Part print with two shaded views. Sizes in mm from the minimum x, y, z corner. A direction names the side the tool comes from. Give positions to 0.01 mm unless a question says otherwise; leave off trailing zeros. Loops run counter-clockwise (first coordinate to the right, second up) from the corner with the lowest first, then second, coordinate; pieces in that order, holes last. Notation, with made-up numbers: M 44.25,-0.75 L 72.25,-0.75 A21 cw 72.25,4.25 Z; hole C 43.25,23 d10. An arc over 180 degrees is marked long. Answer in a Markdown table with one row per item.
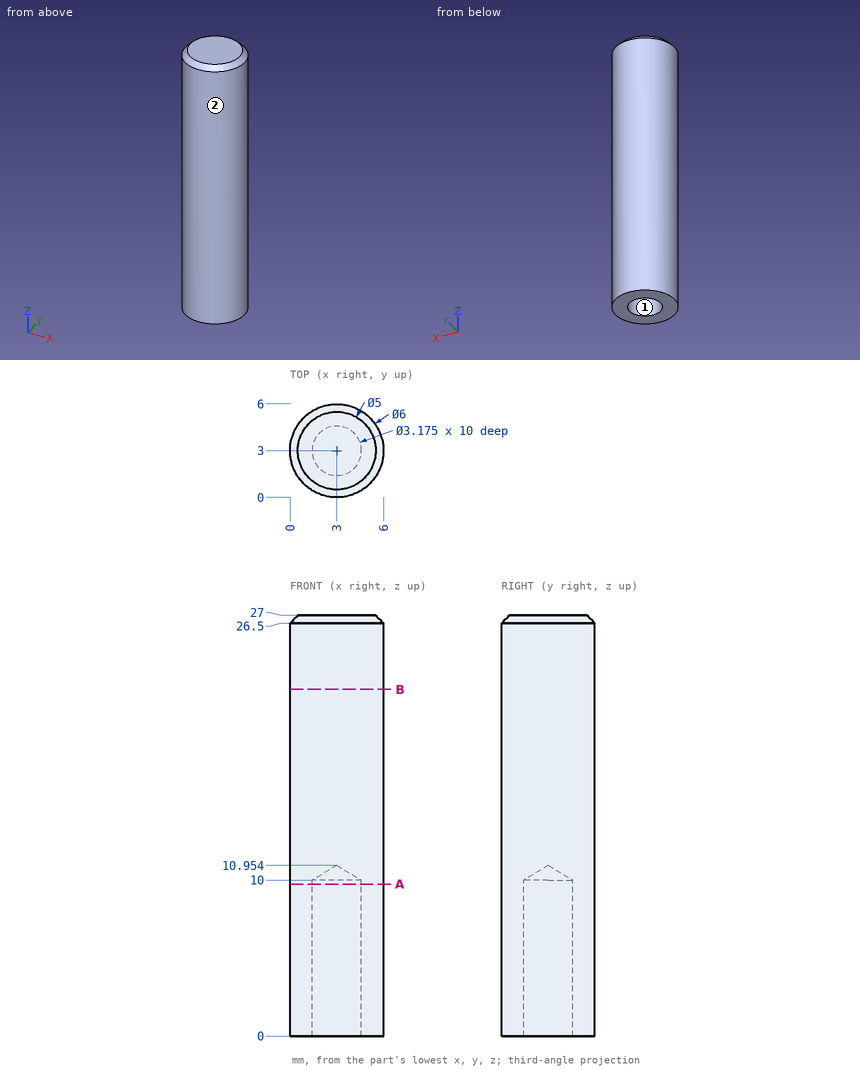
Q1. Probe probe 1 along X at (y, z) = (3.1, 8); probe 2 along Y at (x, z) = (3, 3); probe 3 along X at (y, z) = (2.85, 18.75). List the from-to ranges inside material, lowest first.
Reported:
| item | result |
|---|---|
| probe 1 | 0 to 1.42, 4.58 to 6 |
| probe 2 | 0 to 1.41, 4.59 to 6 |
| probe 3 | 0 to 6 |
Q2. Saw through at B-B (z = 22.25). Give the cut face in (x, y).
Reported:
| item | result |
|---|---|
| outline | C 3,3 d6 |
Q3. 3-axis set-ups, long thin cutter, end or side, ignore diameter. For the marked faces 1 and 2: which of +Z, -Z, +X, -X, +Y, -Y reach the whole face in a straight line?
Reported:
| item | result |
|---|---|
| face 1 | -Z |
| face 2 | +Z, -Z |
Q4. Drop flat-ended pins along their axis: pin 1 (1.5 mm diameter, centred on x = 2, z = 9.5, fed in from +Y); pin 2 (1.5 mm diameter, centred on x = 3.5, y = 3.5, fed in from -Z); pin 3 (1.5 mm diameter, centred on y = 4, z = 9.5, fed in from -X). Give the stop position or say it passes through.
Reported:
| item | result |
|---|---|
| pin 1 | y = 5.99 |
| pin 2 | z = 10.08 |
| pin 3 | x = 0.01 |
Q5. Saw through at A-A (z = 9.75). Give the cut face in (x, y) (1 decimal).
Reported:
| item | result |
|---|---|
| outline | C 3,3 d6; hole C 3,3 d3.2 |
